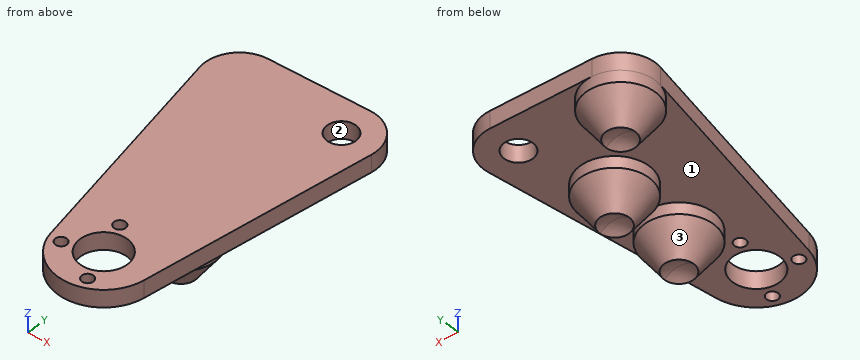
from build123d import *

# Parameters (mm, degrees)
BOSS_EXTRUDE1_DEPTH = 3
BOSS_EXTRUDE5_DEPTH = 3
SKETCH3_R           = 4.1
CUT_EXTRUDE1_DEPTH  = 50
BOSS_EXTRUDE2_START = -7
SKETCH1_3_R         = 6
BOSS_EXTRUDE2_DEPTH = 7
SKETCH1_4_R         = 6
BOSS_EXTRUDE3_DEPTH = 7
SKETCH1_5_R         = 6
BOSS_EXTRUDE6_DEPTH = 7
CHAMFER8_SIZE       = 5
CHAMFER8_SIZE_2     = 3.501037691
SKETCH9_R           = 1
CUT_EXTRUDE3_DEPTH  = 3
SKETCH13_R          = 2.5
CUT_EXTRUDE4_DEPTH  = 3


with BuildPart() as part:
    # Sketch1 → Boss-Extrude1 (new body)
    with BuildSketch(Plane.XY):
        with BuildLine():
            Line((8.47879639, 27.808299752), (-6.041521678, 42.809946731))
            ThreePointArc((-6.041521678, 42.809946731), (-13.178830457, 43.929795654), (-16.218713498, 37.375838886))
            Line((-16.218713498, 37.375838886), (-7.821268925, -1.68159222))
            ThreePointArc((-7.821268925, -1.68159222), (0.48240993, -7.985441795), (7.966824047, -0.727814955))
            Line((7.966824047, -0.727814955), (10.142674299, 23.089524856))
            ThreePointArc((10.142674299, 23.089524856), (9.826089659, 25.630630372), (8.47879639, 27.808299752))
        make_face()
    extrude(amount=BOSS_EXTRUDE1_DEPTH)

    # Sketch10 → Boss-Extrude5 (add)
    with BuildSketch(Plane.XY):
        with BuildLine():
            Line((-6.041521678, 42.809946731), (8.47879639, 27.808299752))
            ThreePointArc((8.47879639, 27.808299752), (9.826089659, 25.630630372), (10.142674299, 23.089524856))
            Line((10.142674299, 23.089524856), (7.966824047, -0.727814955))
            ThreePointArc((7.966824047, -0.727814955), (7.953555222, -0.86078995), (7.938067055, -0.993524752))
            Line((7.938067055, -0.993524752), (12.899477398, 38.647166557))
            ThreePointArc((12.899477398, 38.647166557), (11.356622336, 43.459959023), (6.684210782, 45.38659945))
            Line((6.684210782, 45.38659945), (-10.614478128, 44.631322381))
            ThreePointArc((-10.614478128, 44.631322381), (-8.13262373, 44.211168584), (-6.041521678, 42.809946731))
        make_face()
    extrude(amount=BOSS_EXTRUDE5_DEPTH)

    # Sketch3 → Cut-Extrude1 (cut)
    with BuildSketch(Plane.XY.offset(3)):
        Circle(SKETCH3_R)
    extrude(amount=-CUT_EXTRUDE1_DEPTH, mode=Mode.SUBTRACT)

    # Sketch1<3> → Boss-Extrude2 (add)
    with BuildSketch(Plane.XY.offset(BOSS_EXTRUDE2_START)):
        with Locations(Location((-10.352761804, 38.637033052, 0), (0, 0, 192.134016017))):
            Circle(SKETCH1_3_R)
    extrude(amount=BOSS_EXTRUDE2_DEPTH)

    # Sketch1<4> → Boss-Extrude3 (add)
    with BuildSketch(Plane.XY):
        with Locations((2.167556264, 25.701683368)):
            Circle(SKETCH1_4_R)
    extrude(amount=-BOSS_EXTRUDE3_DEPTH)

    # Sketch1<5> → Boss-Extrude6 (add)
    with BuildSketch(Plane.XY):
        with Locations((2.25742631, 12.802500789)):
            Circle(SKETCH1_5_R)
    extrude(amount=-BOSS_EXTRUDE6_DEPTH)

    # Sketch6 one side → Cut-Revolve1 (revolve, cut)
    with BuildSketch(Plane(origin=(-10.352761804, 0, 0), x_dir=(0, 0, -1), z_dir=(1, 0, 0))):
        with BuildLine():
            ThreePointArc((10, 34.637033052), (12.828427125, 35.808605927), (14, 38.637033052))
            ThreePointArc((14, 38.637033052), (12.828427125, 41.465460176), (10, 42.637033052))
            Line((10, 42.637033052), (10, 34.637033052))
        make_face()
    revolve(axis=Axis((-10.352761804, 42.637033052, -10), (0, -1, 0)), mode=Mode.SUBTRACT)

    # Sketch7 one side → Cut-Revolve2 (revolve, cut)
    with BuildSketch(Plane(origin=(2.167556264, 0, 0), x_dir=(0, 0, -1), z_dir=(1, 0, 0))):
        with BuildLine():
            ThreePointArc((10, 21.701683368), (12.828427125, 22.873256243), (14, 25.701683368))
            ThreePointArc((14, 25.701683368), (12.828427125, 28.530110493), (10, 29.701683368))
            Line((10, 29.701683368), (10, 21.701683368))
        make_face()
    revolve(axis=Axis((2.167556264, 29.701683368, -10), (0, -1, 0)), mode=Mode.SUBTRACT)

    # Sketch14 one side → Cut-Revolve3 (revolve, cut)
    with BuildSketch(Plane(origin=(2.25742631, 0, 0), x_dir=(0, 0, -1), z_dir=(1, 0, 0))):
        with BuildLine():
            ThreePointArc((10, 8.802500789), (12.828427125, 9.974073664), (14, 12.802500789))
            ThreePointArc((14, 12.802500789), (12.828427125, 15.630927914), (10, 16.802500789))
            Line((10, 16.802500789), (10, 8.802500789))
        make_face()
    revolve(axis=Axis((2.25742631, 16.802500789, -10), (0, -1, 0)), mode=Mode.SUBTRACT)

    # Chamfer8
    # the kernel refuses this chamfer: 5, 3.501037691 mm, written as the material it takes off along each edge
    with BuildSketch(Plane(origin=(-10.352761804, 38.637033052, -7), x_dir=(-0.9776586156884893, -0.21019902751931718, 0), z_dir=(-0.21019902751931718, 0.9776586156884893, 0))) as chamfer8_piece_1:
        Polygon((6, CHAMFER8_SIZE), (6 - CHAMFER8_SIZE_2, 0), (6, 0), align=None)
    revolve(axis=Axis((-10.352761804, 38.637033052, -7), (0, 0, 1)), mode=Mode.SUBTRACT)
    with BuildSketch(Plane(origin=(2.167556264, 25.701683368, -7), x_dir=(1, 0, 0), z_dir=(0, -1, 0))) as chamfer8_piece_2:
        Polygon((6, CHAMFER8_SIZE), (6 - CHAMFER8_SIZE_2, 0), (6, 0), align=None)
    revolve(axis=Axis((2.167556264, 25.701683368, -7), (0, 0, 1)), mode=Mode.SUBTRACT)
    with BuildSketch(Plane(origin=(2.25742631, 12.802500789, -7), x_dir=(1, 0, 0), z_dir=(0, -1, 0))) as chamfer8_piece_3:
        Polygon((6, CHAMFER8_SIZE), (6 - CHAMFER8_SIZE_2, 0), (6, 0), align=None)
    revolve(axis=Axis((2.25742631, 12.802500789, -7), (0, 0, 1)), mode=Mode.SUBTRACT)

    # Sketch9 → Cut-Extrude3 (cut)
    with BuildSketch(Plane.XY.offset(3)):
        with Locations((-2.135535698, 5.607092587)):
            Circle(SKETCH9_R)
        with Locations((2.135535698, -5.607092587)):
            Circle(SKETCH9_R)
        with Locations((-5.607092587, -2.135535698)):
            Circle(SKETCH9_R)
    extrude(amount=-CUT_EXTRUDE3_DEPTH, mode=Mode.SUBTRACT)

    # Sketch13 → Cut-Extrude4 (cut)
    with BuildSketch(Plane.XY.offset(3)):
        with Locations((6.945927107, 39.39231012)):
            Circle(SKETCH13_R)
    extrude(amount=-CUT_EXTRUDE4_DEPTH, mode=Mode.SUBTRACT)


solid = part.part
Geometry: final body of the model. Coordinates: model frame, mm. Face numbers are marked on the shaded views. Coordinates: 2 decimals unless noted, no trailing zeros. Order: outer loops, then holes, each group sorted by start corner. A loop starts at its lowest first (then second) coordinate and runs counter-clockwise, first axis right, second up.
(1) Draft query along X for the marked faces 1, 2 and 3. Return one class per face: pulls with the +X half, pulls with the -X half, needs draft (parallel to the pull), parting line crosses it, or undercut.
(2) Section query A-A (y = 0). Return the cut outline in (x, z).
(3) First-contact query: pin 1 (5 mm diameter, centred on x = 4, z = 1, fed in from -Y); pin 2 (1.2 mm diameter, centred on x = -2.14, y = 5.61, fed in from +Z); pin 3 (2 mm diameter, centred on x = -8, y = 16.5, fed in from -Z). Flat tips, straight axial feed; report the tip coordinate or a pass-through.
(4) Section query B-B (x = -2.5). State how many separate pieces and enclosed holes the cut face has, plus the area to 3 significant figures.
(5) Material intervals for probe 1 along Y at (x, z) = (1.75, -6.5); probe 2 along Y at (x, z) = (2.25, 2.25); probe 3 along Z at (x, y) = (8.5, 8.5), sorted ascending.
Solution:
1. face 1: needs draft
1. face 2: undercut
1. face 3: parting line crosses it
2. outline: (-8.18, 0) - (-4.1, 0) - (-4.1, 3) - (-8.18, 3) - close; (4.1, 0) - (8.06, 0) - (8.06, 3) - (4.1, 3) - close
3. pin 1: stops at y = -7.86
3. pin 2: passes through
3. pin 3: stops at z = 0
4. separate pieces: 3
4. enclosed holes: 0
4. area: 180 mm2
5. probe 1: y = 10 to 10.93, 14.67 to 15.61, 22.88 to 23.81, 27.59 to 28.52
5. probe 2: y = -7.68 to -6.6, -4.61 to -3.43, 3.43 to 45.19
5. probe 3: z = 0 to 3
